```python
from build123d import *

# Parameters (mm, degrees)
PAD001_DEPTH    = 2
SKETCH002_R     = 3
SKETCH002_R_2   = 4.9
PAD002_DEPTH    = 8
CHAMFER_SIZE    = 1
CHAMFER001_SIZE = 1
PAD003_DEPTH    = 9
PAD004_DEPTH    = 6
PAD005_DEPTH    = 8.5
PAD006_DEPTH    = 0.4


with BuildPart() as part:
    # Sketch001 → Pad001 (new body)
    with BuildSketch(Plane.XY):
        with BuildLine():
            Line((-21.73, 22.75), (21.73, 22.75))
            ThreePointArc((22.75, 21.73), (22.451249, 22.451249), (21.73, 22.75))
            Line((22.75, 21.73), (22.75, -15.25))
            ThreePointArc((15.25, -22.75), (20.553301, -20.553301), (22.75, -15.25))
            Line((15.25, -22.75), (-15.25, -22.75))
            ThreePointArc((-22.75, -15.25), (-20.553301, -20.553301), (-15.25, -22.75))
            Line((-22.75, -15.25), (-22.75, 21.73))
            ThreePointArc((-21.73, 22.75), (-22.451249, 22.451249), (-22.75, 21.73))
        make_face()
    extrude(amount=PAD001_DEPTH)

    # Sketch002 → Pad002 (join)
    with BuildSketch(Plane.XY):
        with Locations((-18.05, 18.05)):
            Circle(SKETCH002_R)
        with Locations((18.05, 18.05)):
            Circle(SKETCH002_R)
        with Locations((6.2, -18.15)):
            Circle(SKETCH002_R)
        with Locations((-6.2, -18.15)):
            Circle(SKETCH002_R)
        with Locations((15.8, -16.15)):
            Circle(SKETCH002_R_2)
    extrude(amount=-PAD002_DEPTH)

    # Chamfer
    chamfer_edges = [part.edges().sort_by_distance(p)[0] for p in [
        (15.05, 18.05, -8),
        (-21.05, 18.05, -8),
        (-9.2, -18.15, -8),
        (3.2, -18.15, -8),
        (10.9, -16.15, -8),
    ]]
    chamfer(chamfer_edges, length=CHAMFER_SIZE)

    # Chamfer001
    chamfer001_edges = [part.edges().sort_by_distance(p)[0] for p in [
        (0, -22.75, 2),
    ]]
    chamfer(chamfer001_edges, length=CHAMFER001_SIZE)

    # Sketch003 → Pad003 (join, symmetric)
    with BuildSketch(Plane.XZ.offset(-3)):
        with BuildLine():
            ThreePointArc((-20.8, -0.965685), (-20.677375, -0.349207), (-21.2, 0))
            Line((-21.2, 0), (-15.2, 0))
            ThreePointArc((-15.2, 0), (-16.381381, -0.386204), (-17.106508, -1.395661))
            Line((-19.2, -8), (-17.106508, -1.395661))
            Line((-20.8, -8), (-19.2, -8))
            Line((-21.4, -6.255228), (-20.8, -8))
            Line((-20.8, -5.655228), (-21.4, -6.255228))
            Line((-21.4, -3.910457), (-20.8, -5.655228))
            Line((-20.8, -3.310457), (-21.4, -3.910457))
            Line((-21.4, -1.565685), (-20.8, -3.310457))
            Line((-20.8, -0.965685), (-21.4, -1.565685))
        make_face()
        with BuildLine():
            Line((3, 0), (9, 0))
            ThreePointArc((9, 0), (8.477375, -0.349207), (8.6, -0.965685))
            Line((8.6, -0.965685), (9.2, -1.565685))
            Line((9.2, -1.565685), (8.6, -3.310457))
            Line((8.6, -3.310457), (9.2, -3.910457))
            Line((9.2, -3.910457), (8.6, -5.655228))
            Line((8.6, -5.655228), (9.2, -6.255228))
            Line((9.2, -6.255228), (8.6, -8))
            Line((8.6, -8), (7, -8))
            Line((7, -8), (4.906508, -1.395661))
            ThreePointArc((4.906508, -1.395661), (4.181381, -0.386204), (3, 0))
        make_face()
    extrude(amount=PAD003_DEPTH, both=True)

    # Sketch004 → Pad004 (join, symmetric)
    with BuildSketch(Plane.YZ):
        with BuildLine():
            ThreePointArc((-20.8, -1.023773), (-20.665406, -0.381157), (-21.2, 0))
            Line((-21.2, 0), (-15.2, 0))
            ThreePointArc((-15.2, 0), (-16.381381, -0.386204), (-17.106508, -1.395661))
            Line((-19.2, -8), (-17.106508, -1.395661))
            Line((-20.8, -8), (-19.2, -8))
            Line((-21.4, -6.274591), (-20.8, -8))
            Line((-20.8, -5.674591), (-21.4, -6.274591))
            Line((-21.4, -3.949182), (-20.8, -5.674591))
            Line((-20.8, -3.349182), (-21.4, -3.949182))
            Line((-21.4, -1.623773), (-20.8, -3.349182))
            Line((-20.8, -1.023773), (-21.4, -1.623773))
        make_face()
    extrude(amount=PAD004_DEPTH, both=True)

    # Sketch005 → Pad005 (join, symmetric)
    with BuildSketch(Plane.YZ.offset(-5)):
        with BuildLine():
            Line((15.2, 0), (21.2, 0))
            ThreePointArc((21.2, 0), (20.665406, -0.381157), (20.8, -1.023773))
            Line((20.8, -1.023773), (21.4, -1.623773))
            Line((21.4, -1.623773), (20.8, -3.349182))
            Line((20.8, -3.349182), (21.4, -3.949182))
            Line((21.4, -3.949182), (20.8, -5.674591))
            Line((20.8, -5.674591), (21.4, -6.274591))
            Line((21.4, -6.274591), (20.8, -8))
            Line((20.8, -8), (19.2, -8))
            Line((19.2, -8), (17.106508, -1.395661))
            ThreePointArc((17.106508, -1.395661), (16.381381, -0.386204), (15.2, 0))
        make_face()
    extrude(amount=PAD005_DEPTH, both=True)

    # Sketch006 → Pad006 (new body)
    with BuildSketch(Plane(origin=(0, 0, 0), x_dir=(-1, 0, 0), z_dir=(0, 0, 1))):
        Polygon((8.162951, -4.789), (8.162951, 4.722677), (6.260616, 4.722677), (6.260616, -3.158427), (1.640658, -3.158427), (1.640658, -4.789), align=None)
    extrude(amount=-PAD006_DEPTH)


solid = part.part
```
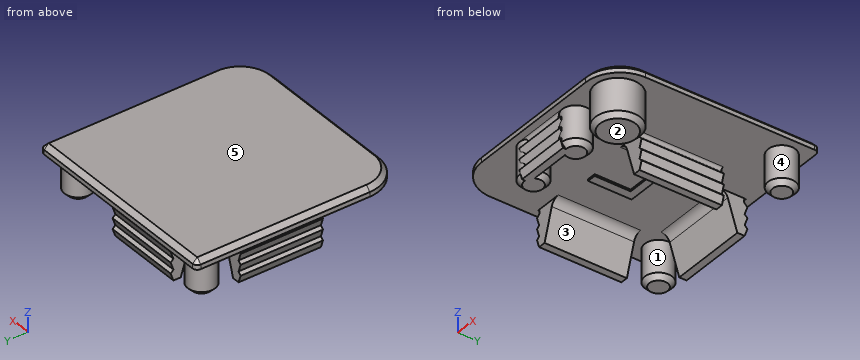
Model file for the job. Use its own axes, mm. Face numbers are marked on the shaded views. A direction names the side the tool comes from. Give positions to 0.01 mm unless a question says otherwise; leave off trailing zeros. Loops run counter-clockwise (first coordinate to the right, second up) from the corner with the lowest first, then second, coordinate; pieces in that order, holes last. Notation, with made-up numbers: (-11, 70) - (24, 70) arc R19 cw to (24, 94) - close; hole circle Ø9 at (72.25, 82.5). An arc over 180 degrees is marked (long way). One line per item, written item: value. Start each with the question number.
1. Pin check, flat tips, straight feed: pin 1 (3 mm diameter, centred on x = 6, z = -3, fed in from +Y); pin 2 (3.5 mm diameter, centred on x = -6, y = -1.5, fed in from -Z); pin 3 (5 mm diameter, centred on y = -0.5, z = -6, fed in from -X). Stop position of each tip, or through.
2. Slice it at A-A (y = 14). List the corners of the cut face in (x, z).
3. Probe L1, parallel to Z at x = -4, y = -8; L2, parallel to X at y = -18, z = -5; L3, parallel to X at y = 7, z = -5. List the from-to ranges inside material, lowest first. Write a range as from..to.
4. Pull direction Y, two halves, no side cores. Call the marked faces 1 and 2: pulls with the +Y half, pulls with the -Y half, needs draft (parallel to the pull), parting line crosses it, or undercut.
5. Which spindle directions (+Z, -Z, +X, -X, +Y, -Y) get a long thin tool onto all of the face, cutting with end or side? Do the marked faces 3, 4 and 5. Say none if no direction does.
Solution:
1. pin 1: stops at y = 12
1. pin 2: stops at z = -0.4
1. pin 3: stops at x = -21.4
2. outline: (-22.75, 0) - (22.75, 0) - (22.75, 1) - (21.75, 2) - (-21.75, 2) - (-22.75, 1) - close
3. L1: z = 0..2
3. L2: x = -9.2..-3.2, 3.2..9.2, 11.26..20.34
3. L3: x = -21.03..-18.25, 6.05..8.83
4. face 1: undercut
4. face 2: needs draft
5. face 3: -Z, -Y
5. face 4: -Z
5. face 5: +Z, +X, -X, +Y, -Y
